The listing builds one solid part. Answer for the finished solid, in the listing's coordinates (mm). A direction names the side the tool comes from. Coordinates: 2 decimals unless noted, no trailing zeros. Order: outer loops, then holes, each group sorted by start corner. A loop starts at its lowest first (then second) coordinate and runs counter-clockwise, first axis right, second up. Notation, with made-up numbers: (88, -40) -> (116, -40) arc R23 cw to (116, -11) -> close; hole circle Ø2 at (6.5, 61). An arc over 180 degrees is marked (long way). Return JSON: item names as keys, results as strings.
from build123d import *

# Parameters (mm, degrees)
EXTRUDE_1_DEPTH     = 8
CUT_EXTRUDE_START   = -1
SKETCH_3_W          = 2.6
SKETCH_3_H          = 4.7
CUT_EXTRUDE_1_DEPTH = 15
SKETCH_4_R          = 1
CUT_EXTRUDE_2_DEPTH = 27.4
CHAMFER_1_SIZE      = 0.2


with BuildPart() as part:
    # Эскиз2 → Бобышка-Вытянуть1 (new body)
    with BuildSketch(Plane.XY):
        Polygon((21.4, -5), (21.4, 10), (16.4, 10), (16.4, 0), (0, 0), (0, 10), (-5, 10), (-5, -5), align=None)
    extrude(amount=EXTRUDE_1_DEPTH)

    # Эскиз3 → Вырез-Вытянуть1 (cut, through all)
    with BuildSketch(Plane(origin=(0, 10, 0), x_dir=(1, 0, 0), z_dir=(0, 1, 0)).offset(CUT_EXTRUDE_START)):
        with Locations((-2.5, -4)):
            Rectangle(SKETCH_3_W, SKETCH_3_H)
        with Locations((18.9, -4)):
            Rectangle(SKETCH_3_W, SKETCH_3_H)
    extrude(amount=-CUT_EXTRUDE_1_DEPTH, mode=Mode.SUBTRACT)

    # Эскиз4 → Вырез-Вытянуть2 (cut, through all)
    with BuildSketch(Plane(origin=(21.4, 0, 0), x_dir=(0, 0, -1), z_dir=(1, 0, 0))):
        with Locations((-4, 7.5)):
            Circle(SKETCH_4_R)
    extrude(amount=-CUT_EXTRUDE_2_DEPTH, mode=Mode.SUBTRACT)

    # Фаска1
    chamfer_1_edges = [part.edges().sort_by_distance(p)[0] for p in [
        (-1.2, -5, 4),
        (-2.5, -5, 6.35),
        (-3.8, -5, 4),
        (-2.5, -5, 1.65),
        (20.2, -5, 4),
        (18.9, -5, 6.35),
        (17.6, -5, 4),
        (18.9, -5, 1.65),
    ]]
    chamfer(chamfer_1_edges, length=CHAMFER_1_SIZE)


solid = part.part
1. The part is cut by section C-C on z = 7. Give the vertices of the cut face in (x, y).
Answer block:
{"outline": "(-5, -5) -> (21.4, -5) -> (21.4, 10) -> (16.4, 10) -> (16.4, 0) -> (0, 0) -> (0, 10) -> (-5, 10) -> close"}
2. Each of these flat-tipped pins is pushed along its axis until it touches: pin 1 Ø2 at (x, z) = (19, 4) entering from -Y; pin 2 Ø1.5 at (x, z) = (3.5, 4) entering from +Y. Where does it stop, or does it pass through?
Answer block:
{"pin 1": "stops at y = 9", "pin 2": "stops at y = 0"}
3. The part is cut by section B-B on y = 2.75. Give the vertices of the cut face in (x, z).
Answer block:
{"outline": "(-5, 0) -> (0, 0) -> (0, 8) -> (-5, 8) -> close; (16.4, 0) -> (21.4, 0) -> (21.4, 8) -> (16.4, 8) -> close; hole (-3.8, 1.65) -> (-1.2, 1.65) -> (-1.2, 6.35) -> (-3.8, 6.35) -> close; hole (17.6, 1.65) -> (20.2, 1.65) -> (20.2, 6.35) -> (17.6, 6.35) -> close"}
4. For faces 1 (the face through (19, 2, 1.65)), 2 (the face through (8, -1, 0)), 3 (the face through (8, 0, 4)), determine the directions among +Z, -Z, +X, -X, +Y, -Y from which every point of the face is accessible in a straight line to the end or side of a thin tool.
Answer block:
{"face 1": "-Y", "face 2": "-Z, +X, -X, +Y, -Y", "face 3": "+Z, -Z, +Y"}
5. The part is cut by section A-A on y = 7.5. Give the number of separate pieces and of enclosed holes in the cut face, and give its area (3 significant figures).
Answer block:
{"separate pieces": "4", "enclosed holes": "0", "area": "46.0 mm2"}
6. Determine the mould class of faces 4 (the face through (8, -5, 4)), 5 (the face through (-3, 9, 4)), 6 (the face through (-5, 3, 4)) for opening direction X: pulls with the +X half, pulls with the -X half, needs draft (parallel to the pull), parting line crosses it, or undercut.
Answer block:
{"face 4": "needs draft", "face 5": "undercut", "face 6": "pulls with the -X half"}
7. Consider line 1 (X direction, y = -1.25, z = 3.25); line 2 (X direction, y = 5.25, z = 4.75); line 3 (X direction, y = 9.75, z = 2). Determine where each line is inside the solid, lowest interval first. Write a range as from..to.
Answer block:
{"line 1": "x = -5..-3.8, -1.2..17.6, 20.2..21.4", "line 2": "x = -5..-3.8, -1.2..0, 16.4..17.6, 20.2..21.4", "line 3": "x = -5..0, 16.4..21.4"}
